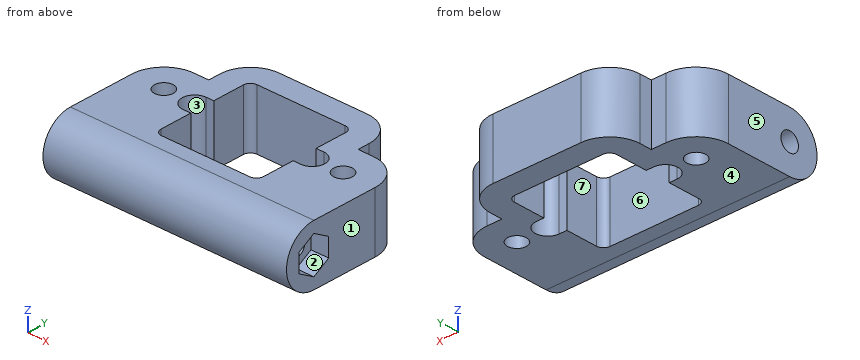
Autodesk Inventor part; units mm, degrees
ref_plane "YZ Plane" through (0, 0, 0) normal (1, 0, 0) x (0, 1, 0)
ref_plane "XZ Plane" through (0, 0, 0) normal (0, 1, 0) x (-1, 0, 0)
ref_plane "XY Plane" through (0, 0, 0) normal (0, 0, 1) x (1, 0, 0)
sketch "Эскиз1" plane through (0, 0, 0) normal (0, 0, 1) x (1, 0, 0)
  line L0 (16.51, 16.51) -> (0, 16.51)
  line L1 (0, 16.51) -> (0, 11.176)
  line L2 (0, 11.176) -> (-6.731, 11.176)
  line L3 (-6.731, 11.176) -> (-7.4684, 11.0622)
  line L4 (-7.4684, 11.0622) -> (-8.1512, 10.7614)
  line L5 (-8.1512, 10.7614) -> (-8.733, 10.2942)
  line L6 (-8.733, 10.2942) -> (-9.1739, 9.6923)
  line L7 (-9.1739, 9.6923) -> (-9.4441, 8.9967)
  line L8 (-9.4441, 8.9967) -> (-9.525, 8.255)
  line L9 (-9.525, 8.255) -> (-9.4441, 7.5133)
  line L10 (-9.4441, 7.5133) -> (-9.1739, 6.8177)
  line L11 (-9.1739, 6.8177) -> (-8.733, 6.2158)
  line L12 (-8.733, 6.2158) -> (-8.1512, 5.7486)
  line L13 (-8.1512, 5.7486) -> (-7.4684, 5.4478)
  line L14 (-7.4684, 5.4478) -> (-6.731, 5.334)
  line L15 (-6.731, 5.334) -> (0, 5.334)
  line L16 (0, 5.334) -> (0, 0)
  line L17 (0, 0) -> (16.51, 0)
  line L18 (16.51, 0) -> (16.51, 5.334)
  line L19 (16.51, 5.334) -> (23.241, 5.334)
  line L20 (23.241, 5.334) -> (23.9784, 5.4478)
  line L21 (23.9784, 5.4478) -> (24.6612, 5.7486)
  line L22 (24.6612, 5.7486) -> (25.243, 6.2158)
  line L23 (25.243, 6.2158) -> (25.6839, 6.8177)
  line L24 (25.6839, 6.8177) -> (25.9541, 7.5133)
  line L25 (25.9541, 7.5133) -> (26.035, 8.255)
  line L26 (26.035, 8.255) -> (25.9541, 8.9967)
  line L27 (25.9541, 8.9967) -> (25.6839, 9.6923)
  line L28 (25.6839, 9.6923) -> (25.243, 10.2942)
  line L29 (25.243, 10.2942) -> (24.6612, 10.7614)
  line L30 (24.6612, 10.7614) -> (23.9784, 11.0622)
  line L31 (23.9784, 11.0622) -> (23.241, 11.176)
  line L32 (23.241, 11.176) -> (16.51, 11.176)
  line L33 (16.51, 11.176) -> (16.51, 16.51)
  circle A0 centre (18.26, 8.26) radius 1.27
  circle A1 centre (-1.75, 8.26) radius 1.27
  circle A2 centre (11.505, 9.45) radius 0.127
  circle A3 centre (8.386, 9.267) radius 0.127
  circle A4 centre (4.826, 15.748) radius 0.127
  circle A5 centre (4.191, 15.748) radius 0.127
  circle A6 centre (-6.985, 8.255) radius 1.5
  circle A7 centre (23.495, 8.255) radius 1.5
  circle A8 centre (3.048, 4.445) radius 0.1651
  circle A9 centre (6.985, 4.445) radius 0.1651
  circle A10 centre (2.286, 6.731) radius 0.2032
  circle A11 centre (13.716, 8.509) radius 0.2032
  circle A12 centre (12.319, 1.778) radius 0.2032
  circle A13 centre (15.367, 16.002) radius 0.2032
  circle A14 centre (14.732, 1.778) radius 0.2032
  circle A15 centre (13.462, 1.778) radius 0.2032
  circle A16 centre (11.5062, 15.748) radius 0.127
  circle A17 centre (7.874, 15.748) radius 0.127
  circle A18 centre (3.429, 14.859) radius 0.127
  circle A19 centre (14.478, 15.113) radius 0.1651
  circle A20 centre (2.286, 10.541) radius 0.2032
  circle A21 centre (13.716, 11.176) radius 0.2032
  circle A22 centre (5.505, 15.748) radius 0.127
  circle A23 centre (14.478, 14.224) radius 0.1651
  circle A24 centre (13.462, 15.113) radius 0.1651
  circle A25 centre (10.414, 15.7988) radius 0.127
  circle A26 centre (5.005, 9.727) radius 0.127
  circle A27 centre (6.8072, 8.636) radius 0.127
  circle A28 centre (4.699, 8.382) radius 0.127
  circle A29 centre (10.922, 8.636) radius 0.127
  circle A30 centre (6.378, 16.129) radius 0.127
  circle A31 centre (10.4648, 5.4864) radius 0.127
  circle A32 centre (11.2268, 5.4864) radius 0.127
  circle A33 centre (10.4648, 6.1214) radius 0.127
  circle A34 centre (9.1948, 7.8994) radius 0.127
  circle A35 centre (2.955, 14.2) radius 0.3
  circle A36 centre (9.779, 15.748) radius 0.127
  circle A37 centre (9.906, 8.636) radius 0.127
  circle A38 centre (9.194, 7.112) radius 0.127
  circle A39 centre (9.144, 15.748) radius 0.127
  circle A40 centre (5.588, 7.874) radius 0.127
  circle A41 centre (13.335, 6.096) radius 0.1651
  circle A42 centre (6.8072, 7.874) radius 0.127
  circle A43 centre (6.878, 15.748) radius 0.127
  circle A44 centre (7.378, 16.141) radius 0.127
  circle A45 centre (5.588, 7.239) radius 0.127
  circle A46 centre (8.509, 15.748) radius 0.127
  circle A47 centre (7.5946, 7.1186) radius 0.127
  circle A48 centre (13.555, 14.2) radius 0.3
  line L34 (9.655, 16.755) -> (9.655, 15.8775)
  arc A49 (6.855, 15.8775) -> (9.655, 15.8775) centre (8.255, 8.255) ccw
  line L35 (6.855, 15.8775) -> (6.855, 16.755)
  line L36 (6.855, 16.755) -> (0.755, 16.755)
  arc A50 (0.755, 16.755) -> (-0.245, 15.755) centre (0.755, 15.755) ccw
  line L37 (-0.245, 15.755) -> (-0.245, 10.155)
  line L38 (-0.245, 10.155) -> (-1.745, 10.155)
  arc A51 (-1.745, 10.155) -> (-1.745, 6.355) centre (-1.745, 8.255) ccw
  line L39 (-1.745, 6.355) -> (-0.245, 6.355)
  line L40 (-0.245, 6.355) -> (-0.245, 0.755)
  arc A52 (-0.245, 0.755) -> (0.755, -0.245) centre (0.755, 0.755) ccw
  line L41 (0.755, -0.245) -> (15.755, -0.245)
  arc A53 (15.755, -0.245) -> (16.755, 0.755) centre (15.755, 0.755) ccw
  line L42 (16.755, 0.755) -> (16.755, 6.355)
  line L43 (16.755, 6.355) -> (18.255, 6.355)
  arc A54 (18.255, 6.355) -> (18.255, 10.155) centre (18.255, 8.255) ccw
  line L44 (18.255, 10.155) -> (16.755, 10.155)
  line L45 (16.755, 10.155) -> (16.755, 15.755)
  arc A55 (16.755, 15.755) -> (15.755, 16.755) centre (15.755, 15.755) ccw
  line L46 (15.755, 16.755) -> (9.655, 16.755)
  circle A56 centre (-1.745, 8.255) radius 0.9
  circle A57 centre (18.255, 8.255) radius 0.9
  line L47 (-1.745, 10.355) -> (-0.445, 10.355)
  line L48 (-0.445, 10.355) -> (-0.445, 15.755)
  arc A58 (0.755, 16.955) -> (-0.445, 15.755) centre (0.755, 15.755) ccw
  line L49 (0.755, 16.955) -> (7.055, 16.955)
  line L50 (7.055, 16.955) -> (7.055, 15.709)
  arc A59 (7.055, 15.709) -> (9.455, 15.709) centre (8.255, 8.255) ccw
  line L51 (9.455, 15.709) -> (9.455, 16.955)
  line L52 (9.455, 16.955) -> (15.755, 16.955)
  arc A60 (16.955, 15.755) -> (15.755, 16.955) centre (15.755, 15.755) ccw
  line L53 (16.955, 15.755) -> (16.955, 10.355)
  line L54 (16.955, 10.355) -> (18.255, 10.355)
  arc A61 (18.255, 6.155) -> (18.255, 10.355) centre (18.255, 8.255) ccw
  line L55 (18.255, 6.155) -> (16.955, 6.155)
  line L56 (16.955, 6.155) -> (16.955, 0.755)
  arc A62 (15.755, -0.445) -> (16.955, 0.755) centre (15.755, 0.755) ccw
  line L57 (15.755, -0.445) -> (0.755, -0.445)
  arc A63 (-0.445, 0.755) -> (0.755, -0.445) centre (0.755, 0.755) ccw
  line L58 (-0.445, 0.755) -> (-0.445, 6.155)
  line L59 (-0.445, 6.155) -> (-1.745, 6.155)
  arc A64 (-1.745, 10.355) -> (-1.745, 6.155) centre (-1.745, 8.255) ccw
  line L60 (7.055, 16.955) -> (9.455, 16.955)
  line L61 (7.055, 20.955) -> (0.755, 20.955)
  arc A65 (0.755, 20.955) -> (-4.445, 15.755) centre (0.755, 15.755) ccw
  line L62 (-4.445, 15.755) -> (-4.445, 13.7249)
  line L63 (-4.445, 2.7851) -> (-4.445, 0.755)
  line L64 (20.955, 0.755) -> (20.955, 2.7851)
  line L65 (20.955, 13.7249) -> (20.955, 15.755)
  arc A66 (20.955, 15.755) -> (15.755, 20.955) centre (15.755, 15.755) ccw
  line L66 (15.755, 20.955) -> (9.455, 20.955)
  line L67 (7.055, 20.955) -> (9.455, 20.955)
  circle A67 centre (23.495, 8.255) radius 5.4699
  circle A68 centre (-6.985, 8.255) radius 5.4699
  line L68 (-6.985, 13.7249) -> (-4.445, 13.7249)
  line L69 (-4.445, 2.7851) -> (-6.985, 2.7851)
  line L70 (20.955, 2.7851) -> (23.495, 2.7851)
  line L71 (20.955, 13.7249) -> (23.495, 13.7249)
  circle A69 centre (-6.985, 8.255) radius 1.6
  circle A70 centre (23.495, 8.255) radius 1.6
  line L72 (-4.445, 0.755) -> (20.955, 0.755)
  line L73 (20.955, -5.445) -> (-4.445, -5.445)
  line L74 (28.9649, 8.255) -> (28.9649, -5.445)
  line L75 (28.9649, -5.445) -> (-12.4549, -5.445)
  line L76 (-12.4549, -5.445) -> (-12.4549, 8.255)
  point P0 (-0.445, 0.755)
  point P1 (-4.445, -5.445)
  dimension "d0" = 0.2
  dimension "d1" = 4
  dimension "d2" = 3.2
  dimension "d3" = 3.2
extrude "Выдавливание1" add sketch "Эскиз1" along normal blind 10 contours L60 L49 A58 L48 L2 A68 L68 L62 A65 L61 L67 L66 A66 L65 L71 A67 L32 L53 A60 L52 | L32 A67 A61 L54 L53 | A67 L19 L20 L21 L22 L23 L24 L25 L26 L27 L28 L29 L30 L31 L32 | L32 L31 L30 L29 L28 L27 L26 L25 L24 L23 L22 L21 L20 L19 A67 A61 | L74 L75 L73 L76 A68 L69 L63 L72 A63 L57 A62 L64 L70 A67 | A67 L19 L56 L55 A61 | L48 L47 A64 A68 L2 | L70 L64 L72 L56 L19 A67 | A68 A64 L15 L14 L13 L12 L11 L10 L9 L8 L7 L6 L5 L4 L3 L2 | L2 L3 L4 L5 L6 L7 L8 L9 L10 L11 L12 L13 L14 L15 A68 | A64 L59 L58 L15 A68 | L72 L63 L69 A68 L15 L58
sketch "Эскиз3" plane through (-12.4549, -5.445, 0) normal (-1, 0, 0) x (0, 0, 1)
  line L0 (0, 0) -> (0, 13.7)
  line L1 (0, 5) -> (10, 5)
  line L2 (0, 0) -> (10, 0)
  line L3 (10, 0) -> (10, 5)
  line L4 (10, 5) -> (0, 5)
  line L5 (0, 5) -> (0, 0)
  line L6 (5, 5) -> (5, 0)
  line L7 (0, 0) -> (10, 0)
  circle A0 centre (5, 2.5) radius 1.6
  circle A1 centre (5, 2.5) radius 5
  line L8 (10, 0) -> (10, 13.7)
  point P0 (0, 5.445)
  point P1 (0.6699, 0)
  point P2 (0, 2.5)
  point P3 (10, 2.5)
  point P4 (9.3301, 0)
  dimension "d11" = 3.2
extrude "Выдавливание3" cut sketch "Эскиз3" against normal up to surface (41.4198 mm away) contours L0 A1 L2 | A1 L3 L2 | A0 L6 | L6 A0
sketch "Эскиз4" plane through (-12.4549, -5.445, 0) normal (-1, 0, 0) x (0, 0, 1)
  circle A0 centre (5, 2.5) radius 1.6
  circle A1 centre (5, 2.5) radius 5
  line L0 (10, 0) -> (10, 13.7)
  arc A2 (0, 2.5) -> (0.6699, 0) centre (5, 2.5) ccw
  line L1 (0.6699, 0) -> (9.3301, 0)
  line L2 (0.6699, 0) -> (9.3301, 0)
  point P0 (0, 5.445)
extrude "Выдавливание4" add sketch "Эскиз4" against normal up to surface (41.4198 mm away) contours A1 L1 picked at (4.43, -1.3536)
sketch "Эскиз5" plane through (28.9649, 8.255, 10) normal (1, 0, 0) x (0, 0, -1)
  line L0 (5, -11.2) -> (5, -8.5)
  line L1 (6.5588, -8.5) -> (8.1177, -11.2)
  line L2 (8.1177, -11.2) -> (6.5588, -13.9)
  line L3 (6.5588, -13.9) -> (3.4412, -13.9)
  line L4 (3.4412, -13.9) -> (1.8823, -11.2)
  line L5 (1.8823, -11.2) -> (3.4412, -8.5)
  line L6 (3.4412, -8.5) -> (6.5588, -8.5)
  dimension "d17" = 2.7
extrude "Выдавливание5" cut sketch "Эскиз5" against normal blind 3
properties part number "ramka"
Part model, mm, in its own coordinate system. Face numbers are marked on the shaded views. A direction names the side the tool comes from. Round coordinates to 2 decimals unless told otherwise and drop trailing zeros. Loops run counter-clockwise (first coordinate to the right, second up) from the corner with the lowest first, then second, coordinate; pieces in that order, holes last. Notation, with made-up numbers: (14.25, 24) - (69.25, 24) arc R24 cw to (69.25, 49) - close; hole circle Ø10 at (-22.5, 9.25). An arc over 180 degrees is marked (long way). Answer as a JSON object with one key per item and string values.
Item 1: Pin check, flat tips, straight feed: pin 1 (2.5 mm diameter, centred on y = 13, z = 5.5, fed in from -X); pin 2 (2.5 mm diameter, centred on y = -3, z = 5.5, fed in from +X); pin 3 (1 mm diameter, centred on x = -1, z = 4, fed in from -Y). Stop position of each tip, or through.
Output:
{"pin 1": "x = -11.19", "pin 2": "x = 25.96", "pin 3": "y = -7.92"}
Item 2: Tool access for the marked faces 1, 2 and 3: list every direction of +Z, -Z, +X, -X, +Y, -Y with a clear straight run to the whole face (end or side of a thin tool).
Output:
{"face 1": "+Z, -Z, +X, +Y, -Y", "face 2": "+X", "face 3": "+Z, -Z"}
Item 3: Band-saw the part on C-C on z = 5. State how many separate pieces and enclosed holes the cut face has, plus the area to 3 significant figures.
Output:
{"separate pieces": "2", "enclosed holes": "3", "area": "575 mm2"}
Item 4: Wall check: L1, parallel to Y at x = 13, z = 5 (3 decimals); L2, parallel to X at y = 7.75, z = 1.25; L3, parallel to X at y = 15.5, z = 3.5 (3 decimals). Give the ranges that are in metal, low to high.
Output:
{"L1": "-7.945 to -4.545, -1.345 to -0.445, 16.955 to 20.955", "L2": "-12.45 to -8.5, -5.47 to -3.78, 20.29 to 21.98, 25.01 to 28.96", "L3": "-4.445 to -0.445, 16.955 to 20.955"}
Item 5: Band-saw the part on A-A on x = 5. List the corners of the cut face in (y, z) (3 decimals), plus the area to 3 significant figures.
Output:
{"outline": "(-2.945, 0) - (-0.445, 0) - (-0.445, 10) - (-2.945, 10) arc R5 ccw to start; (16.955, 0) - (20.955, 0) - (20.955, 10) - (16.955, 10) - close; hole circle Ø3.2 at (-2.945, 5)", "area": "96.2 mm2"}
Item 6: Band-saw the part on B-B on y = 4.75. List the corners of the cut face in (x, z) (3 decimals), plus the area to 3 significant figures.
Output:
{"outline": "(-12.455, 0) - (-0.445, 0) - (-0.445, 10) - (-12.455, 10) - close; (16.955, 0) - (28.965, 0) - (28.965, 10) - (16.955, 10) - close", "area": "240 mm2"}
Item 7: Pull direction X, two halves, no side cores. Call the marked faces 4, 5, 6 and 7: pulls with the +X half, pulls with the -X half, needs draft (parallel to the pull), parting line crosses it, or undercut.
Output:
{"face 4": "needs draft", "face 5": "pulls with the -X half", "face 6": "undercut", "face 7": "undercut"}
